Source: CAD feature listing. Evaluate the final solid. Frame: model axes, mm. Face numbers are marked on the shaded views. A direction names the side the tool comes from. Give positions to 0.01 mm unless a question says otherwise; leave off trailing zeros. Write each loop counter-clockwise with the first axis right and the second up, starting at its lowest first coordinate (ties: lowest second). Pieces come first, ordered by that corner, then holes. Notation, with made-up numbers: (74.25, 23.25) -> (79.25, 23.25) arc R29 cw to (79.25, 43.25) -> close; hole circle Ø4 at (46, 1.25). An arc over 180 degrees is marked (long way). Answer as a JSON object with one key per item and string values. Group by question number.
Item 1: Section query B-B on y = 21. Return the cut outline in (x, z).
Item 2: Section query A-A on z = 2. Return the cut outline in (x, y).
Item 3: First-contact query: pin 1 Ø1 at (y, z) = (19, 11) entering from +X; pin 2 Ø3.5 at (x, z) = (15, 4.5) entering from -Y; pin 3 Ø1.5 at (y, z) = (19.5, 1.5) entering from -X. Flat tips, straight axial feed; report the tip coordinate or a pass-through.
Item 4: Section query D-D on z = 11.25. Return the cut outline in (x, y), plus the area to 3 significant figures.
Item 5: Access query for the marked faces 4 and 5. Directions: +Z, -Z, +X, -X, +Y, -Y. A direction counts if a zero-diameter tool reaches every point of the face in a straight line with its end or side. Return the directions, or none.
Item 6: Ray query, probe 1 along X at (y, z) = (9.25, 6.25); probe 2 along X at (y, z) = (13, 2.5); probe 3 along Y at (x, z) = (6, 2.75). Return the intervals inside material, ascending. Write a range as from..to.
Item 7: Section query C-C on x = 15.25. Return the cut outline in (y, z), plus the area to 3 significant figures.
Item 8: Pull-direction query (Y, two-part tool) for the marked faces 1, 2 and 3; classes: pulls with the +Y half, pulls with the -Y half, needs draft (parallel to the pull), parting line crosses it, or undercut.
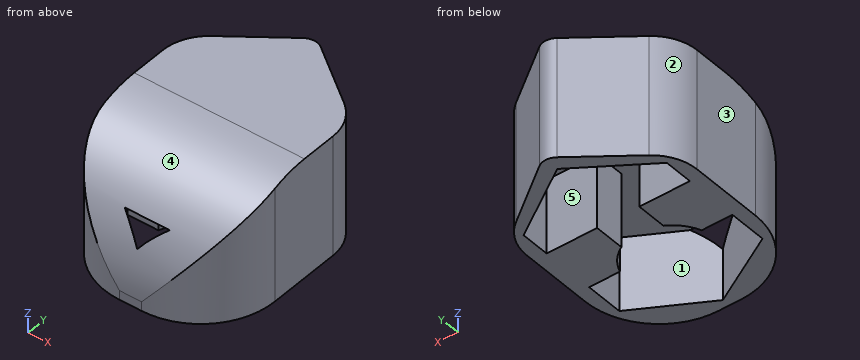
from build123d import *

# Parameters (mm, degrees)
BOSS_EXTRUDE1_DEPTH = 13
FILLET1_R           = 12
CUT_EXTRUDE1_DEPTH  = 8
SKETCH5_R           = 4.716803238
CUT_EXTRUDE2_DEPTH  = 8
SKETCH6_W           = 4.554767644
SKETCH6_H           = 3.613594083
CUT_EXTRUDE3_DEPTH  = 8


with BuildPart() as part:
    # Sketch2 → Boss-Extrude1 (new body)
    with BuildSketch(Plane.XY):
        with BuildLine():
            Line((8, 0), (10.4, 0))
            ThreePointArc((10.4, 0), (16.056854249, 2.343145751), (18.4, 8))
            Line((18.4, 8), (18.4, 15.886901909))
            ThreePointArc((18.4, 15.886901909), (17.867444955, 18.132327386), (16.383225769, 19.899427797))
            Line((16.383225769, 19.899427797), (10.154632246, 24.530251678))
            ThreePointArc((10.154632246, 24.530251678), (9.2, 24.846243393), (8.245367754, 24.530251678))
            Line((8.245367754, 24.530251678), (2.016774231, 19.899427797))
            ThreePointArc((2.016774231, 19.899427797), (0.532555045, 18.132327386), (0, 15.886901909))
            Line((0, 15.886901909), (0, 8))
            ThreePointArc((0, 8), (2.343145751, 2.343145751), (8, 0))
        make_face()
    extrude(amount=BOSS_EXTRUDE1_DEPTH)

    # Fillet1
    # the kernel refuses this fillet: 12 mm, written as the material it takes off along each edge
    with BuildSketch(Plane(origin=(-22, 0, 13), x_dir=(0, 0, -1), z_dir=(1, 0, 0))) as fillet1_piece_1:
        with BuildLine():
            CenterArc((FILLET1_R, FILLET1_R), FILLET1_R, 180, 90)
            Line((0, FILLET1_R), (0, 0))
            Line((0, 0), (FILLET1_R, 0))
        make_face()
    extrude(amount=62.4, mode=Mode.SUBTRACT)

    # Sketch4 → Cut-Extrude1 (cut)
    with BuildSketch(Plane(origin=(0, 0, 0), x_dir=(-1, 0, 0), z_dir=(0, 0, -1))):
        Polygon((-9.2, 23.296502957), (-16.939792645, 18.15947244), (-16.939792645, 15.04300726), (-1.460207355, 15.04300726), (-1.460207355, 18.15947244), align=None)
        Polygon((-1.460207355, 9.289533082), (-16.939792645, 9.289533082), (-16.939792645, 5.214155538), (-9.2, 0.899049904), (-1.460207355, 5.214155538), align=None)
    extrude(amount=-CUT_EXTRUDE1_DEPTH, mode=Mode.SUBTRACT)

    # Sketch5 → Cut-Extrude2 (cut)
    with BuildSketch(Plane(origin=(0, 0, 0), x_dir=(-1, 0, 0), z_dir=(0, 0, -1))):
        with Locations((-9.2, 7.64)):
            Circle(SKETCH5_R)
    extrude(amount=-CUT_EXTRUDE2_DEPTH, mode=Mode.SUBTRACT)

    # Sketch6 → Cut-Extrude3 (cut)
    with BuildSketch(Plane(origin=(0, 0, 0), x_dir=(-1, 0, 0), z_dir=(0, 0, -1))):
        with Locations((-9.2, 13.577384858)):
            Rectangle(SKETCH6_W, SKETCH6_H)
    extrude(amount=-CUT_EXTRUDE3_DEPTH, mode=Mode.SUBTRACT)


solid = part.part
Worked answers:
{
 "1": {"outline": "(3.5, 0) -> (5.74, 0) -> (5.74, 8) -> (12.66, 8) -> (12.66, 0) -> (14.9, 0) -> (14.9, 13) -> (3.5, 13) -> close"},
 "2": {"outline": "(0, 8) arc R8 ccw to (7.18, 0.04) -> (11.22, 0.04) arc R8 ccw to (18.4, 8) -> (18.4, 15.89) arc R5 ccw to (16.38, 19.9) -> (10.15, 24.53) arc R1.6 ccw to (8.25, 24.53) -> (2.02, 19.9) arc R5 ccw to (0, 15.89) -> close; hole (1.46, 5.21) -> (9.2, 0.9) -> (16.94, 5.21) -> (16.94, 9.29) -> (13.62, 9.29) arc R4.72 ccw to (11.48, 11.77) -> (11.48, 15.04) -> (16.94, 15.04) -> (16.94, 18.16) -> (9.2, 23.3) -> (1.46, 18.16) -> (1.46, 15.04) -> (6.92, 15.04) -> (6.92, 11.77) arc R4.72 ccw to (4.78, 9.29) -> (1.46, 9.29) -> close"},
 "3": {"pin 1": "x = 17.66", "pin 2": "y = 0.52", "pin 3": "x = 0.9"},
 "4": {"outline": "(0, 8) arc R8 ccw to (0.32, 5.76) -> (18.08, 5.76) arc R8 ccw to (18.4, 8) -> (18.4, 15.89) arc R5 ccw to (16.38, 19.9) -> (10.15, 24.53) arc R1.6 ccw to (8.25, 24.53) -> (2.02, 19.9) arc R5 ccw to (0, 15.89) -> close", "area": "293 mm^2"},
 "5": {"face 4": "+Z, +X, -X, -Y", "face 5": "-Z"},
 "6": {"probe 1": "0..1.46, 16.94..18.4", "probe 2": "0..6.92, 11.48..18.4", "probe 3": "0.25..2.68, 11.11..15.04, 21.17..22.86"},
 "7": {"outline": "(1.64, 0) -> (4.27, 0) -> (4.27, 8) -> (9.29, 8) -> (9.29, 0) -> (15.04, 0) -> (15.04, 8) -> (19.28, 8) -> (19.28, 0) -> (20.74, 0) -> (20.74, 13) -> (12, 13) arc R12 ccw to (1.64, 7.05) -> close", "area": "156 mm^2"},
 "8": {"face 1": "undercut", "face 2": "pulls with the +Y half", "face 3": "needs draft"}
}
